Model file for the job. Use its own axes, mm. Face numbers are marked on the shaded views. A direction names the side the tool comes from. Give positions to 0.01 mm unless a question says otherwise; leave off trailing zeros. Order: outer loops, then holes, each group sorted by start corner. A loop starts at its lowest first (then second) coordinate and runs counter-clockwise, first axis right, second up. Notation, with made-up numbers: (-20, 40) - (-15, 40) arc R23 cw to (-15, 75) - close; hole circle Ø10 at (28.5, 48.25). An arc over 180 degrees is marked (long way). Use CSV: the item, a comma, the result in double quotes. Start each with the question number.
(1) Drop flat-ended pins along their axis: pin 1 Ø2 at (x, z) = (18, 6.5) entering from +Y; pin 2 Ø1 at (y, z) = (5, 10) entering from -X; pin 3 Ø1 at (y, z) = (4, 11) entering from +X. Give the stop position or say it passes through.
(2) Tool access for the marked faces 1 and 2: list every direction of +Z, -Z, +X, -X, +Y, -Y with a clear straight run to the whole face (end or side of a thin tool).
(3) Band-saw the part on A-A, the plane z = 10. Give the cut face in (x, y).
(4) Probe L1, parallel to X at y = 0.35, z = 10; L2, parallel to Y at x = 16.5, z = 5.75. List the from-to ranges inside material, lowest first.
(5) Band-saw the part on D-D, the plane y = 2.5. Give the cut face in (x, z).
(6) Band-saw the part on B-B, the plane x = 22.5. Give the cut face in (y, z), then the cut area to 4 significant figures.
(7) Band-saw the part on C-C, the plane z = 16.5. Give the cut face in (x, y).
from build123d import *

# Parameters (mm, degrees)
EXTRU_MINCE1_DEPTH      = 20
ESQUISSE2_R             = 1.75
ENL_V_MAT_EXTRU_1_DEPTH = 45.544921147
ESQUISSE3_W             = 1.5
ESQUISSE3_H             = 14
ENL_V_MAT_EXTRU_2_DEPTH = 46.171893916
CONG_1_R                = 2


with BuildPart() as part:
    # Esquisse1 → Extru.-Mince1 (new body)
    with BuildSketch(Plane.XY):
        Polygon((0, 19.5), (0, 0), (35.5, 0), (35.5, 1.5), (1.5, 1.5), (1.5, 19.5), align=None)
    extrude(amount=EXTRU_MINCE1_DEPTH)

    # Esquisse2 → Enlèv. mat.-Extru.1 (cut, through all)
    with BuildSketch(Plane(origin=(0, 1.5, 0), x_dir=(1, 0, 0), z_dir=(0, 1, 0))):
        with Locations(Location((22.5, -10, 0), (0, 0, 270))):
            Circle(ESQUISSE2_R)
    extrude(amount=-ENL_V_MAT_EXTRU_1_DEPTH, mode=Mode.SUBTRACT)

    # Esquisse3 → Enlèv. mat.-Extru.2 (cut, through all)
    with BuildSketch(Plane.XY.offset(20)):
        with Locations((0.75, 12.5)):
            Rectangle(ESQUISSE3_W, ESQUISSE3_H)
    extrude(amount=-ENL_V_MAT_EXTRU_2_DEPTH, mode=Mode.SUBTRACT)

    # Congé1
    cong_1_edges = [part.edges().sort_by_distance(p)[0] for p in [
        (0.75, 5.5, 0),
        (0.75, 5.5, 20),
        (35.5, 0.75, 0),
        (35.5, 0.75, 20),
    ]]
    fillet(cong_1_edges, radius=CONG_1_R)


solid = part.part
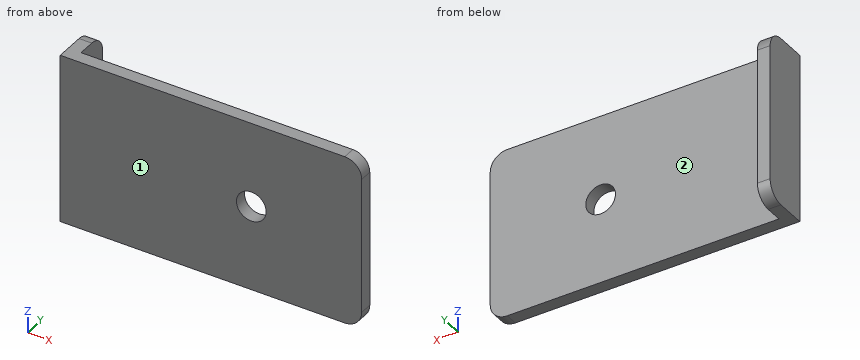
Answer block:
1,pin 1,"stops at y = 1.5"
1,pin 2,"stops at x = 0"
1,pin 3,"stops at x = 1.5"
2,face 1,"+Z, -Z, +X, -X, -Y"
2,face 2,"+Z, -Z, +X, +Y"
3,outline,"(0, 0) - (20.75, 0) - (20.75, 1.5) - (1.5, 1.5) - (1.5, 5.5) - (0, 5.5) - close; (24.25, 0) - (35.5, 0) - (35.5, 1.5) - (24.25, 1.5) - close"
4,L1,"x = 0 to 20.75, 24.25 to 35.5"
4,L2,"y = 0 to 1.5"
5,outline,"(0, 0) - (1.5, 0) - (1.5, 20) - (0, 20) - close"
6,outline,"(0, 0) - (1.5, 0) - (1.5, 8.25) - (0, 8.25) - close; (0, 11.75) - (1.5, 11.75) - (1.5, 20) - (0, 20) - close"
6,area,"24.75 mm2"
7,outline,"(0, 0) - (35.5, 0) - (35.5, 1.5) - (1.5, 1.5) - (1.5, 5.5) - (0, 5.5) - close"
